Check sheet for the modelled part. Datum: model origin and axes. Units: mm. Face numbers are marked on the shaded views. A direction names the side the tool comes from. Give positions to 0.01 mm unless a question says otherwise; leave off trailing zeros. Write each loop counter-clockwise with the first axis right and the second up, starting at its lowest first coordinate (ties: lowest second). Pieces come first, ordered by that corner, then holes. Notation, with made-up numbers: (32.5, 75.25) -> (63.5, 75.25) arc R23 ccw to (63.5, 89.25) -> close; hole circle Ø8 at (60.5, 75). An arc over 180 degrees is marked (long way). Answer as a JSON object with one key per item and string values.
from build123d import *

# Parameters (mm, degrees)
F2_R     = 0.25
F3_DEPTH = 25


with BuildPart() as f1:
    # F0 (on Top) → F1 (revolve)
    with BuildSketch(Plane.XY):
        with BuildLine():
            Line((0, -2), (0, 0.403768))
            ThreePointArc((0, 0.403768), (-1.42086, 0.302312), (-2.812888, 0))
            Line((-2.812888, 0), (-5, 0))
            Line((-5, 0), (-5, -0.738022))
            Line((-5, -0.738022), (-2.802643, -0.738022))
            Line((-2.802643, -0.738022), (-1.151906, -1.127067))
            Line((-1.151906, -1.127067), (-1.151906, -2))
            Line((-1.151906, -2), (0, -2))
        make_face()
    revolve(axis=Axis((0, -0.798116, 0), (0, 1, 0)))

    # F2 (on face) → F3 (cut)
    with BuildSketch(Plane.XZ.offset(0.738022)):
        with Locations((3, 3)):
            Circle(F2_R)
        with Locations((-3, 3)):
            Circle(F2_R)
        with Locations((-3, -3)):
            Circle(F2_R)
        with Locations((3, -3)):
            Circle(F2_R)
    extrude(amount=-F3_DEPTH, mode=Mode.SUBTRACT)


solid = f1.part
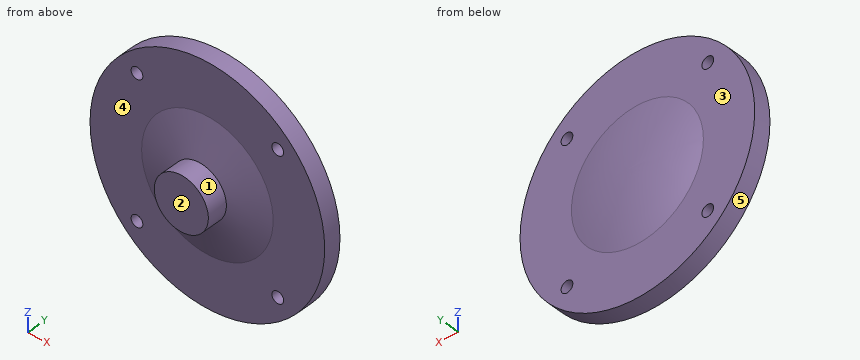
1. Go/stop test with flat-tipped pins: P1, Ø5, axis at x = 2, z = 1.5, coming from the +Y side; P2, Ø2, axis at x = -2, z = 3.5, coming from the +Y side; P3, Ø1, axis at x = -2, z = -1.5, coming from the -Y side. Record where each tip stops, or that it passes through.
Determined:
{"P1": "y = 0.4", "P2": "y = 0", "P3": "y = -0.93"}
2. Sectioned sample at C-C, the plane z = 3.75. Enter the section's corners in (x, y), plus the area to 3 significant figures.
Determined:
{"outline": "(-3.31, -0.74) -> (3.31, -0.74) -> (3.31, 0) -> (-3.31, 0) -> close", "area": "4.88 mm^2"}
3. Access from +Z, -Z, +X, -X, +Y, -Y to the whole of each face (thin tool, end or side, straight path). Record for the marked faces 1 and 2.
Determined:
{"face 1": "-Y", "face 2": "+Z, -Z, +X, -X, -Y"}
4. Sectioned sample at B-B, the plane y = -0.3. Enter the section's corners in (x, z).
Determined:
{"outline": "circle Ø10 at (0, 0); hole circle Ø0.5 at (-3, -3); hole circle Ø0.5 at (-3, 3); hole circle Ø0.5 at (3, -3); hole circle Ø0.5 at (3, 3)"}
5. Sectioned sample at A-A, the plane x = 3. Enter the section's corners in (y, z).
Determined:
{"outline": "(-0.74, -4) -> (0, -4) -> (0, -3.25) -> (-0.74, -3.25) -> close; (-0.74, -2.75) -> (0, -2.75) -> (0, 2.75) -> (-0.74, 2.75) -> close; (-0.74, 3.25) -> (0, 3.25) -> (0, 4) -> (-0.74, 4) -> close"}
6. Scan lines: L1, parallel to Z at x = 3, y = -0.15; L2, parallel to Z at x = 0, y = -1.65; L3, parallel to Y at x = -4.5, z = 1.25. Record each from-to range of solid material in increasing order. Write a range as [from, to].
Determined:
{"L1": "[-4, -3.25], [-2.75, 2.75], [3.25, 4]", "L2": "[-1.15, 1.15]", "L3": "[-0.74, 0]"}
7. Mould release check, pull along Y, two halves, no side actions. Record for the marked faces 3, 4 and 5: released by +Y, released by -Y, zero draft, split by the parting line, or undercut.
Determined:
{"face 3": "released by +Y", "face 4": "released by -Y", "face 5": "zero draft"}
